Check sheet for the modelled part. Datum: model origin and axes. Units: mm. A direction names the side the tool comes from. Give positions to 0.01 mm unless a question says otherwise; leave off trailing zeros. Loops run counter-clockwise (first coordinate to the right, second up) from the corner with the lowest first, then second, coordinate; pieces in that order, holes last. Notation, with made-up numbers: (18, 9.25) -> (25, 9.25) arc R17 ccw to (25, 40.25) -> close; hole circle Ø9 at (-31.75, -19). An arc over 180 degrees is marked (long way). Write each question's results on one line, items separated by ' | '. Start each with the question number.
Item 1: Cross-section at D-D on y = 77.5. Enter the section's corners in (x, z).
Item 2: Scan lines: line 1 along X through (y, z) = (23, -66.5); line 2 along Z through (x, y) = (97, 33.5); line 3 along X through (y, z) = (100, -93). Record each from-to range of solid material in increasing order.
Item 3: Gauge pin test, flat ends, axial feed: pin 1 Ø6 at (x, z) = (59.5, -4.5) entering from +Y; pin 2 Ø3.5 at (y, z) = (90.34, -81.76) entering from +X; pin 3 Ø6 at (x, y) = (116, 51.5) entering from -Z. Record the tip position at first contact, or that the pin passes through.
Item 4: Access from +Z, -Z, +X, -X, +Y, -Y to the whole of each face (thin tool, end or side, straight path). Record for faces 4 (the face through (6, 50.8, 0)), 5 (the face through (75, 60, 101.6)), 6 (the face through (75, 12.7, -5)).
Item 5: Cross-section at A-A on z = -49. Enter the section's corners in (x, y).
Item 6: Mould release check, pull along X, two halves, no side actions. Record for faces 1 (the face through (152.4, 50, 1)), 2 (the face through (10, 20, 19.207)), 3 (the face through (12.7, 54, -5)): pulls with the +X half, pulls with the -X half, needs draft (parallel to the pull), parting line crosses it, or undercut.
Item 7: Cross-section at C-C on x = 21.5. Enter the section's corners in (y, z), then the cut area to 3 significant figures.
Item 8: Cross-section at B-B on y = 35.5. Enter the section's corners in (x, z).
from build123d import *

# Parameters (mm, degrees)
F1_DEPTH       = 101.6
F3_T           = -12.7
F2_W           = 50.8
F2_H           = 38.1
F4_DEPTH       = 25.4
F7_D           = 4
F7_DEPTH       = 14.2
F7_CSINK_D     = 6.72
F7_CSINK_ANGLE = 90
F7_TIP         = 1.2017212381


with BuildPart() as f1:
    # F0 (on Top) → F1 (new body, symmetric)
    with BuildSketch(Plane.XY):
        Polygon((0, 101.6), (0, 0), (152.4, 0), (152.4, 101.6), (76.2, 152.4), align=None)
    extrude(amount=F1_DEPTH, both=True)

    # F3
    f3_openings = [f1.faces().sort_by_distance(p)[0] for p in [
        (76.2, 64.346667, -101.6),
    ]]
    offset(amount=F3_T, openings=f3_openings)

    # F2 (on face) → F4 (cut)
    with BuildSketch(Plane(origin=(0, 0, 0), x_dir=(0, -1, 0), z_dir=(-1, 0, 0))):
        with Locations((-25.4, 0.1572931677)):
            Rectangle(F2_W, F2_H)
    extrude(amount=-F4_DEPTH, mode=Mode.SUBTRACT)

    # F7
    with Locations(Plane.YZ.offset(152.4)):
        with Locations((88.5495916009, 80.6001722813), (90.3433784842, -81.7593187094)):
            CounterSinkHole(F7_D / 2, F7_CSINK_D / 2, depth=F7_DEPTH, counter_sink_angle=F7_CSINK_ANGLE)
            with Locations((0, 0, -(F7_DEPTH + F7_TIP / 2))):  # 118° drill point
                Cone(0, F7_D / 2, F7_TIP, mode=Mode.SUBTRACT)


solid = f1.part
Answer sheet:
1) outline: (0, -101.6) -> (12.7, -101.6) -> (12.7, 88.9) -> (139.7, 88.9) -> (139.7, -101.6) -> (152.4, -101.6) -> (152.4, 101.6) -> (0, 101.6) -> close
2) line 1: x = 0 to 12.7, 139.7 to 152.4 | line 2: z = 88.9 to 101.6 | line 3: x = 0 to 20.5, 131.9 to 152.4
3) pin 1: stops at y = 143.27 | pin 2: stops at x = 12.7 | pin 3: stops at z = 88.9
4) face 4: -X, -Y | face 5: +Z, +X, -X, +Y, -Y | face 6: -Z
5) outline: (0, 0) -> (152.4, 0) -> (152.4, 101.6) -> (76.2, 152.4) -> (0, 101.6) -> close; hole (12.7, 12.7) -> (139.7, 12.7) -> (139.7, 94.8) -> (76.2, 137.14) -> (12.7, 94.8) -> close
6) face 1: pulls with the +X half | face 2: needs draft | face 3: undercut
7) outline: (0, -101.6) -> (12.7, -101.6) -> (12.7, -18.89) -> (0, -18.89) -> close; (0, 19.21) -> (12.7, 19.21) -> (12.7, 88.9) -> (100.67, 88.9) -> (100.67, -101.6) -> (115.93, -101.6) -> (115.93, 101.6) -> (0, 101.6) -> close | area: 6,320 mm²
8) outline: (0, -101.6) -> (12.7, -101.6) -> (12.7, -18.89) -> (0, -18.89) -> close; (0, 19.21) -> (12.7, 19.21) -> (12.7, 88.9) -> (139.7, 88.9) -> (139.7, -101.6) -> (152.4, -101.6) -> (152.4, 101.6) -> (0, 101.6) -> close
